Design review of the part shown in the three views and the two pictorial views. Dimensions are in mm from the part's minimum x, y and z. Give positions to 0.01 mm unless a question says otherwise; leave off trailing zeros. Order: outer loops, then holes, each group sorted by start corner. A loop starts at its lowest first (then second) coordinate and runs counter-clockwise, first axis right, second up.
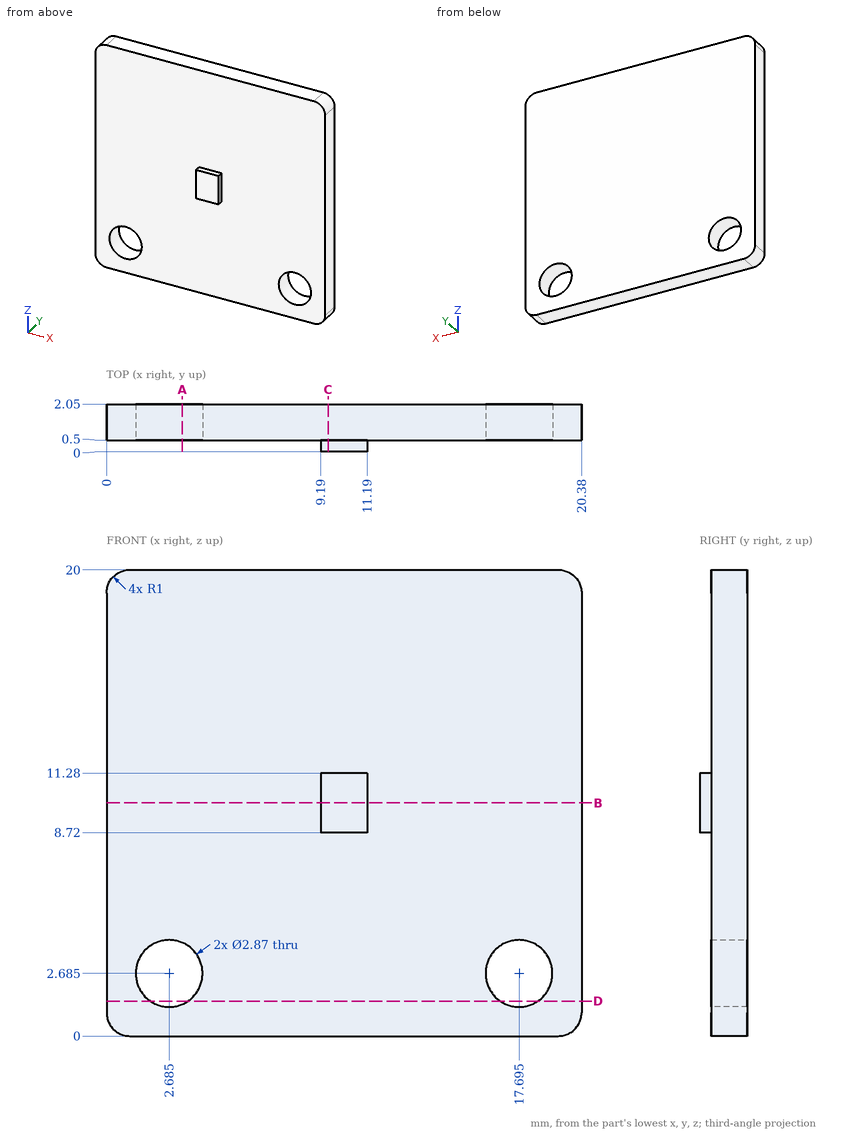
Item 1: Take a section at D-D (z = 1.5). Give the boundary of the cut face in (x, y).
Values found:
outline: (0, 0.5) - (1.88, 0.5) - (1.88, 2.05) - (0, 2.05) - close; (3.49, 0.5) - (16.89, 0.5) - (16.89, 2.05) - (3.49, 2.05) - close; (18.5, 0.5) - (20.38, 0.5) - (20.38, 2.05) - (18.5, 2.05) - close
Item 2: Take a section at A-A (x = 3.25). Give the boundary of the cut face in (y, z).
Values found:
outline: (0.5, 0) - (2.05, 0) - (2.05, 1.37) - (0.5, 1.37) - close; (0.5, 4) - (2.05, 4) - (2.05, 20) - (0.5, 20) - close
Item 3: For line 1 (Y direction, x = 17.5, z = 13.75); line 2 (Z direction, x = 11, y = 0.2), list the stretches that pass through material, from the lowest coordinate up.
Values found:
line 1: y = 0.5 to 2.05
line 2: z = 8.72 to 11.28
Item 4: Take a section at C-C (x = 9.5). Give the boundary of the cut face in (y, z), and give its area (3 significant figures).
Values found:
outline: (0, 8.72) - (0.5, 8.72) - (0.5, 0) - (2.05, 0) - (2.05, 20) - (0.5, 20) - (0.5, 11.28) - (0, 11.28) - close
area: 32.3 mm2
Item 5: Clearance check with flat-ended pins moving along their axes: pin 1 Ø4 at (x, z) = (2.5, 9.5) entering from -Y; pin 2 Ø5 at (x, z) = (9.5, 13) entering from -Y; pin 3 Ø0.6 at (x, y) = (10.5, 0) entering from -Z. State where each tip first meets the part, or that it passes through.
Values found:
pin 1: stops at y = 0.5
pin 2: stops at y = 0
pin 3: stops at z = 8.72
Item 6: Take a section at B-B (z = 10). Give the boundary of the cut face in (x, y), and give its area (3 significant figures).
Values found:
outline: (0, 0.5) - (9.19, 0.5) - (9.19, 0) - (11.19, 0) - (11.19, 0.5) - (20.38, 0.5) - (20.38, 2.05) - (0, 2.05) - close
area: 32.6 mm2
